The drawing under review shows one solid part. Ordinate dimensions are in mm from its lowest x, y, z. A direction names the side the tool comes from. Coordinates: 2 decimals unless noted, no trailing zeros. Order: outer loops, then holes, each group sorted by start corner. A loop starts at its lowest first (then second) coordinate and runs counter-clockwise, first axis right, second up.
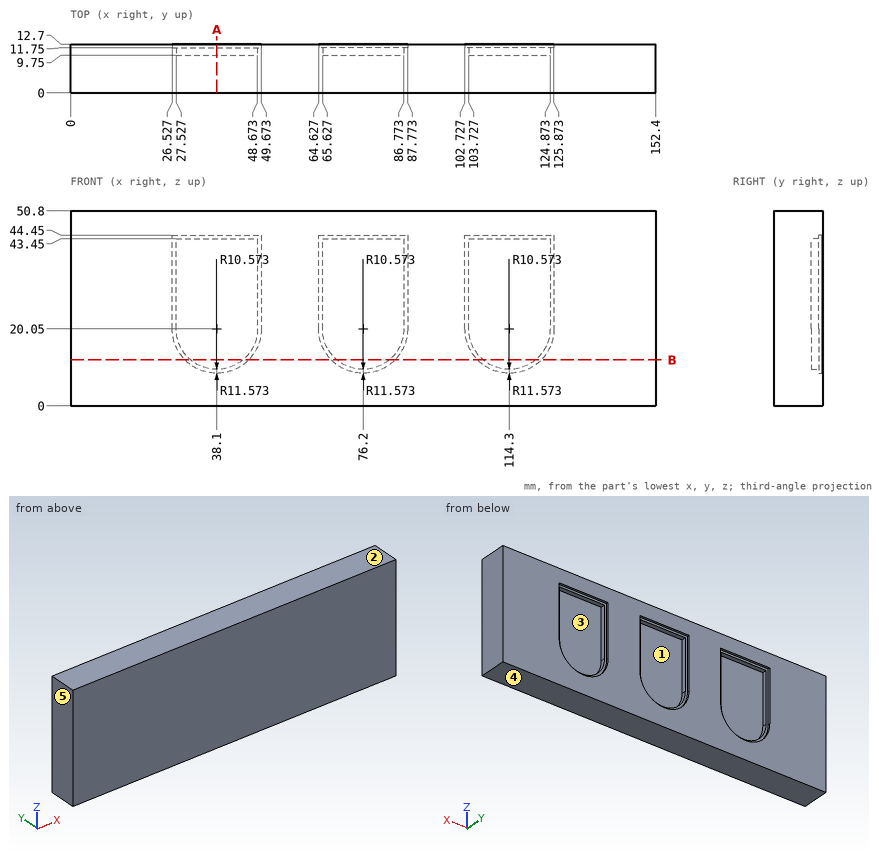
1. Take a section at B-B, the plane z = 12. Give the boundary of the cut face in (x, y).
Answer below:
outline: (0, 0) - (152.4, 0) - (152.4, 12.7) - (122.61, 12.7) - (122.61, 11.75) - (121.15, 11.75) - (121.15, 9.75) - (107.45, 9.75) - (107.45, 11.75) - (105.99, 11.75) - (105.99, 12.7) - (84.51, 12.7) - (84.51, 11.75) - (83.05, 11.75) - (83.05, 9.75) - (69.35, 9.75) - (69.35, 11.75) - (67.89, 11.75) - (67.89, 12.7) - (46.41, 12.7) - (46.41, 11.75) - (44.95, 11.75) - (44.95, 9.75) - (31.25, 9.75) - (31.25, 11.75) - (29.79, 11.75) - (29.79, 12.7) - (0, 12.7) - close
2. Clearance check with a flat-ended pin moving along its axis: pin 1 Ø11.5 at (x, z) = (76.5, 24.5) entering from +Y. State where the tip first meets the part, or that it passes through.
Answer below:
pin 1: stops at y = 9.75
3. Take a section at A-A, the plane x = 38.1. Give the boundary of the cut face in (y, z), plus the area to 3 significant figures.
Answer below:
outline: (0, 0) - (12.7, 0) - (12.7, 8.48) - (11.75, 8.48) - (11.75, 9.48) - (9.75, 9.48) - (9.75, 43.45) - (11.75, 43.45) - (11.75, 44.45) - (12.7, 44.45) - (12.7, 50.8) - (0, 50.8) - close
area: 543 mm2
4. Machinability: for the marked faces 1 and 2, which of the approach directions +Z, -Z, +X, -X, +Y, -Y give a long, thin tool a straight path to every point of the face, cutting with its end or side? Answer none if there is none.
Answer below:
face 1: +Y
face 2: +Z, +X, -X, +Y, -Y
5. The part is to be moulded in two halves that separate along X. For the marked faces 3, 4 and 5, say which applies: +X half, -X half, draft (parallel to the pull), parting line (faces both ways), or undercut.
Answer below:
face 3: undercut
face 4: draft
face 5: -X half
6. To check wall thickness, follow L1, parallel to Y at x = 65, z = 31; L2, parallel to Y at x = 107, z = 31; L3, parallel to Z at x = 66.5, y = 11. State the ranges of each line that lie inside material, in increasing order.
Answer below:
L1: y = 0 to 11.75
L2: y = 0 to 9.75
L3: z = 0 to 15.84, 43.45 to 50.8
